Geometry: final body of the model. Coordinates: model frame, mm. A direction names the side the tool comes from. Round coordinates to 2 decimals unless told otherwise and drop trailing zeros. Order: outer loops, then holes, each group sorted by start corner. A loop starts at its lowest first (then second) coordinate and runs counter-clockwise, first axis right, second up. Notation, with made-up numbers: (69.25, 68.25) -> (78.25, 68.25) arc R18 ccw to (78.25, 82.25) -> close; hole circle Ø2 at (44.25, -6). An arc over 180 degrees is marked (long way). Put each result on its own line as item: value.
```python
from build123d import *

# Parameters (mm, degrees)
SKETCH2_R          = 1.5
CUT_EXTRUDE1_DEPTH = 10
SKETCH3_R          = 2.7
CUT_EXTRUDE2_DEPTH = 2


with BuildPart() as part:
    # Sketch1 → Revolve1 (revolve)
    with BuildSketch(Plane(origin=(0, 0, 0), x_dir=(1, 0, 0), z_dir=(0, 1, 0))):
        Polygon((0, 0), (0, 4.5), (1.8, 4.5), (1.8, 4), (4.8, 4), (4.8, 4.5), (5.5, 4.5), (5.5, 0), align=None)
    revolve(axis=Axis((-92.33576491, 0, 0), (1, 0, 0)))

    # Sketch2 → Cut-Extrude1 (cut)
    with BuildSketch(Plane.ZY):
        Circle(SKETCH2_R)
    extrude(amount=-CUT_EXTRUDE1_DEPTH, mode=Mode.SUBTRACT)

    # Sketch3 → Cut-Extrude2 (cut)
    with BuildSketch(Plane(origin=(5.5, 0, 0), x_dir=(0, 0, -1), z_dir=(1, 0, 0))):
        Circle(SKETCH3_R)
    extrude(amount=-CUT_EXTRUDE2_DEPTH, mode=Mode.SUBTRACT)


solid = part.part
```
1. Set-up query: faces 5 (the face through (4.8, -3, -3)), 6 (the face through (5.5, -3, 0)), 7 (the face through (4.514, -2.636, 0.585)). Return all of +Z, -Z, +X, -X, +Y, -Y with unobstructed straight access to the full face (end or side cutting, diameter ignored); none if empty.
Ans:
face 5: none
face 6: +Z, -Z, +X, +Y, -Y
face 7: +X
2. Cut plane A-A on y = 0. Return loops of the section in (x, z).
Ans:
outline: (0, -4.5) -> (1.8, -4.5) -> (1.8, -4) -> (4.8, -4) -> (4.8, -4.5) -> (5.5, -4.5) -> (5.5, -2.7) -> (3.5, -2.7) -> (3.5, -1.5) -> (0, -1.5) -> close; (0, 1.5) -> (3.5, 1.5) -> (3.5, 2.7) -> (5.5, 2.7) -> (5.5, 4.5) -> (4.8, 4.5) -> (4.8, 4) -> (1.8, 4) -> (1.8, 4.5) -> (0, 4.5) -> close
3. Material intervals for probe 1 along X at (y, z) = (4, -0.5); probe 2 along Y at (x, z) = (1.15, 0); probe 3 along Y at (x, z) = (4.55, 0), sorted ascending.
Ans:
probe 1: 0 to 1.8, 4.8 to 5.5
probe 2: -4.5 to -1.5, 1.5 to 4.5
probe 3: -4 to -2.7, 2.7 to 4
4. Draft query along X for faces 1 (the face through (0, -2, 0)), 2 (the face through (0.91, 4.46, 0.59)), 3 (the face through (3.5, -1.2, -1.2)), 4 (the face through (1.8, -3, 3)). Return one class per face: +X half, -X half, draft (parallel to the pull), parting line (faces both ways), or undercut.
Ans:
face 1: -X half
face 2: draft
face 3: +X half
face 4: undercut
5. Contact query for flat-ended pins moving along their axis: P1, Ø1, axis at x = 3, z = 2, coming from the +Y side; P2, Ø1, axis at x = 3, z = 2.5, coming from the +Y side; P3, Ø3, axis at x = 2.5, z = 3.5, coming from the +Y side. Output: stop coordinate, or through.
Ans:
P1: y = 3.71
P2: y = 3.46
P3: y = 3.94
6. Cut plane C-C on x = 4.4. Return loops of the section in (y, z), and give its area (3 significant figures).
Ans:
outline: circle Ø8 at (0, 0); hole circle Ø5.4 at (0, 0)
area: 27.4 mm²
7. Cut plane D-D on y = 2.5. Return loops of the section in (x, z), and give its area (3 significant figures).
Ans:
outline: (0, -3.74) -> (1.8, -3.74) -> (1.8, -3.12) -> (4.8, -3.12) -> (4.8, -3.74) -> (5.5, -3.74) -> (5.5, -1.02) -> (3.5, -1.02) -> (3.5, 1.02) -> (5.5, 1.02) -> (5.5, 3.74) -> (4.8, 3.74) -> (4.8, 3.12) -> (1.8, 3.12) -> (1.8, 3.74) -> (0, 3.74) -> close
area: 33.4 mm²
